Autodesk Inventor part; units mm, degrees
ref_plane "Work Plane1" through (0, 0, 22) normal (0, 0, 1) x (1, 0, 0)
ref_plane "Plano de trabajo2" through (0, 0, 54) normal (0, 0, 1) x (1, 0, 0)
ref_plane "YZ Plane" through (0, 0, 0) normal (1, 0, 0) x (0, 1, 0)
sketch "Sketch1" plane through (0, 0, 0) normal (0, 0, 1) x (1, 0, 0)
  circle A0 centre (0, 0) radius 50
  circle A1 centre (0, 0) radius 12.5
  circle A2 centre (0, 0) radius 14.5
  line L0 (-15.5, -15.5) -> (15.5, -15.5) construction
  line L1 (15.5, -15.5) -> (15.5, 15.5) construction
  line L2 (15.5, 15.5) -> (-15.5, 15.5) construction
  line L3 (-15.5, 15.5) -> (-15.5, -15.5) construction
  line L4 (-15.5, -15.5) -> (15.5, 15.5) construction
  line L5 (15.5, -15.5) -> (-15.5, 15.5) construction
  dimension "Diametro" = 100
  dimension "d1" = 25
  dimension "d2" = 2
  dimension "d8" = 31
extrude "Extrusion1" add sketch "Sketch1" along normal blind 7 contours A0 | A2
extrude "Extrusion2" add sketch "Sketch1" along normal blind 100 contours A2
ref_plane "Work Plane1" through (0, 0, 22) normal (0, 0, 1) x (1, 0, 0)
sketch "Sketch2" plane through (0, 0, 22) normal (0, 0, 1) x (1, 0, 0)
  arc A0 (2.5, 24.8747) -> (-2.5, 24.8747) centre (0, 0) ccw
  line L0 (2.5, 24.8747) -> (2.5, 14.2829)
  line L1 (-2.5, 24.8747) -> (-2.5, 14.2829)
  line L2 (0, -70) -> (0, 70)
  circle A1 centre (0, 0) radius 14.5
  point P0 (0, 25)
  dimension "d24" = 5
  dimension "d25" = 25
  dimension "Dedos" = 5
extrude "Extrusion3" add sketch "Sketch2" along normal blind 15 contours L0 A1 L2 A0 | L2 A1 L1 A0
sketch "Sketch3" plane through (0, 0, 0) normal (1, 0, 0) x (0, 1, 0)
  line L0 (25, 37) -> (24.8747, 37)
  line L1 (14.2829, 22) -> (14.5, 22)
  line L2 (25, 22) -> (25, 37)
  line L3 (14.2829, 22) -> (14.2829, 37)
  circle A0 centre (25.74, 29.5) radius 1.5
  line L4 (0, -7.4) -> (0, 44.4)
  point P0 (0, 0)
  point P1 (25, 29.5)
  dimension "d31" = 3
  dimension "d92" = 25.74
fillet "Fillet2" radius 8 1 edges at (0, 25, 22)
pattern_circular "Circular Pattern1" count 4 over 360 about axis through (0, 0, 0) along (0, 0, 1) of "Fillet2", "Extrusion3"
ref_plane "Plano de trabajo2" through (0, 0, 54) normal (0, 0, 1) x (1, 0, 0)
sketch "Boceto4" plane through (0, 0, 54) normal (0, 0, 1) x (1, 0, 0)
  circle A0 centre (0, 0) radius 17.5
  circle A1 centre (0, 0) radius 14.5
  line L0 (4, -23.75) -> (4, -26.75)
  dimension "d54" = 35
extrude "Extrusión5" add sketch "Boceto4" against normal up to surface (47 mm away)
sketch "Boceto5" plane through (0, 0, 37) normal (0, 0, 1) x (0, 1, 0)
  arc A0 (-2.5, -17.3205) -> (2.5, -17.3205) centre (0, 0) ccw
  line L0 (-2.5, -17.3205) -> (-2.5, -24.8747)
  arc A1 (-2.5, -24.8747) -> (2.5, -24.8747) centre (0, 0) ccw
  line L1 (2.5, -24.8747) -> (2.5, -17.3205)
  circle A2 centre (0, 0) radius 14.5
  line L2 (2.5, -17.3205) -> (2.5, -14.2829)
  line L3 (-2.5, -17.3205) -> (-2.5, -14.2829)
extrude "Extrusión6" add sketch "Boceto5" along normal blind 20 contours L3 A2 L2 A0 | A0 L1 A1 L0
fillet "Empalme4" radius 8 1 edges at (25, 0, 57)
pattern_circular "Patrón circular2" count 4 over 360 about axis through (0, 0, 54) along (0, 0, -1) of "Extrusión6", "Empalme4"
chamfer "Chaflán1" distance 2 angle 45 1 edges at (-14.5, 0, 100)
sketch "Boceto6" plane through (0, 0, 7) normal (0, 0, 1) x (1, 0, 0)
  circle A0 centre (0, 0) radius 50
  arc A1 (17.3205, 2.5) -> (2.5, 17.3205) centre (0, 0) ccw construction
  line L0 (0, 0) -> (32.476, 18.75) construction
  arc A2 (17.3205, 2.5) -> (2.5, 17.3205) centre (0, 0) ccw construction
  point P0 (16.25, -6.4952)
  point P1 (16.25, 6.4952)
  point P2 (0, 37.5)
  point P3 (-32.476, 18.75)
  point P4 (-32.476, -18.75)
  point P5 (0, -37.5)
  point P6 (32.476, -18.75)
  point P7 (10.8253, 13.75)
  point P8 (15.1554, 8.75)
  dimension "d73" = 360
  dimension "d91" = 37.5
sketch "Boceto8" plane through (0, 0, 7) normal (0, 0, 1) x (1, 0, 0)
  circle A0 centre (0, 0) radius 17.5
  circle A1 centre (0, 0) radius 50
  circle A2 centre (0, 0) radius 46
  dimension "Espesor" = 4
extrude "Extrusión8" add sketch "Boceto8" along normal blind 6 contours A2
sketch "Boceto9" plane through (2.5, 14.0104, 54) normal (1, 0, 0) x (0, -1, 0)
  line L0 (16.5104, 0) -> (28.2932, 0)
  line L1 (-35.9896, 54) -> (64.0104, 54)
  point P0 (1.4018, 24.5)
  point P1 (22.4018, 0)
  dimension "d124" = 21
  dimension "d125" = 29.5
hole "Agujero4" at (2.5, 12.6086, 29.5) direction (-1, 0, 0) diameter 3.4 depth 5
pattern_circular "Patrón circular3" count 4 over 360 about axis through (0, 0, 54) along (0, 0, -1) of "Agujero4"
sketch "Boceto13" plane through (0, 0, 13) normal (0, 0, 1) x (1, 0, 0)
  point P0 (0, 0)
sketch "Boceto15" plane through (0, 0, 0) normal (0, 0, -1) x (-1, 0, 0)
  circle A0 centre (0, 0) radius 27.5 construction
  point P0 (27.5, 0)
  point P1 (13.75, 23.8157)
  point P2 (-13.75, 23.8157)
  point P3 (-27.5, 0)
  point P4 (-13.75, -23.8157)
  point P5 (13.75, -23.8157)
  dimension "d134" = 55
  dimension "d137" = 360
hole "Agujero8" at (-13.75, -23.8157, 0) at (13.75, -23.8157, 0) at (27.5, 0, 0) at (13.75, 23.8157, 0) at (-13.75, 23.8157, 0) at (-27.5, 0, 0) direction (0, 0, 1) diameter 3.4 end through all
sketch "Boceto16" plane through (0, 0, 0) normal (0, 0, -1) x (-1, 0, 0)
  circle A0 centre (0, 0) radius 32.465
  dimension "d146" = 64.93
extrude "Extrusión10" cut sketch "Boceto16" against normal blind 8
sketch "Boceto18" plane through (0, 0, 0) normal (0, 0, -1) x (-1, 0, 0)
  point P0 (0, 0)
  point P1 (-41.233, 0)
  point P2 (-29.1561, -29.1561)
  point P3 (0, -41.233)
  point P4 (29.1561, -29.1561)
  point P5 (41.233, 0)
  point P6 (29.1561, 29.1561)
  point P7 (0, 41.233)
  point P8 (-29.1561, 29.1561)
  dimension "d162" = 41.233
  dimension "d165" = 360
hole "Agujero10" at (41.233, 0, 0) at (29.1561, -29.1561, 0) at (0, -41.233, 0) at (-29.1561, -29.1561, 0) at (-41.233, 0, 0) at (-29.1561, 29.1561, 0) at (0, 41.233, 0) at (29.1561, 29.1561, 0) direction (0, 0, 1) diameter 2.459 depth 10
sketch "Sketch19" plane through (14.2829, -2.5, 54) normal (0, -1, 0) x (1, 0, 0)
  circle A0 centre (6.7167, -24.5) radius 1.7
  line L0 (3.0377, 0) -> (3.0377, -31.9844)
  line L1 (3.0377, 0) -> (-11.7829, 0)
  point P0 (-14.2829, -54)
  dimension "d174" = 3.4
  dimension "d175" = 3.679
  dimension "d176" = 24.5
hole "Hole11" at (20.9995, -2.5, 29.5) direction (0, 1, 0) diameter 4 depth 5
pattern_circular "Circular Pattern4" count 4 over 360 about axis through (0, 0, 0) along (0, 0, 1) of "Hole11"
sketch "Sketch20" plane through (0, 0, 13) normal (0, 0, 1) x (1, 0, 0)
  circle A0 centre (-27.5, 0) radius 1.7
  circle A1 centre (-13.75, 23.8157) radius 1.7
  circle A2 centre (13.75, 23.8157) radius 1.7
  circle A3 centre (27.5, 0) radius 1.7
  circle A4 centre (13.75, -23.8157) radius 1.7
  circle A5 centre (-13.75, -23.8157) radius 1.7
  circle A6 centre (0, 0) radius 46
  circle A7 centre (0, 0) radius 17.5
  circle A8 centre (0, 0) radius 46
extrude "Extrusion12" cut sketch "Sketch20" along normal up to surface contours A6 | A7
sketch "Sketch21" plane through (0, 0, 13) normal (0, 0, 1) x (1, 0, 0)
  circle A0 centre (0, 0) radius 12.5
  circle A1 centre (-27.5, 0) radius 1.7
  circle A2 centre (-13.75, 23.8157) radius 1.7
  circle A3 centre (13.75, 23.8157) radius 1.7
  circle A4 centre (27.5, 0) radius 1.7
  circle A5 centre (13.75, -23.8157) radius 1.7
  circle A6 centre (-13.75, -23.8157) radius 1.7
  circle A7 centre (0, 0) radius 46
  circle A8 centre (-13.75, 23.8157) radius 1.7
  circle A9 centre (13.75, -23.8157) radius 1.7
extrude "Extrusion13" add sketch "Sketch21" against normal up to surface (5 mm away) contours A2 | A5
equation "\"d24\" = Dedos"
equation "\"d91\" = 0.375 * Diametro"
properties part number "Soporte2" material "Aluminum 7075"
Build history of the part. All positions in model axes, mm. A direction names the side the tool comes from. Round coordinates to 2 decimals unless told otherwise and drop trailing zeros. Write each loop counter-clockwise with the first axis right and the second up, starting at its lowest first coordinate (ties: lowest second). Pieces come first, ordered by that corner, then holes. Notation, with made-up numbers: (-31, -7.75) - (1, -7.75) arc R29 cw to (1, 14.25) - close; hole circle Ø5 at (43.5, -16.5). An arc over 180 degrees is marked (long way). One line per question, with ' | ' between items.
1. Band-saw the part on D-D, the plane y = 14.5. Write the cut outline in (x, z).
Results are:
outline: (-47.85, 0) - (-29.05, 0) - (-29.05, 8) - (29.05, 8) - (29.05, 0) - (47.85, 0) - (47.85, 7) - (43.65, 7) - (43.65, 13) - (-43.65, 13) - (-43.65, 7) - (-47.85, 7) - close
2. Band-saw the part on B-B, the plane x = 0. Write the cut outline in (y, z) (1 decimal).
Results are:
outline: (-50, 0) - (-42.5, 0) - (-42.5, 10) - (-40, 10) - (-40, 0) - (-32.5, 0) - (-32.5, 8) - (-12.5, 8) - (-12.5, 13) - (-46, 13) - (-46, 7) - (-50, 7) - close; (12.5, 8) - (32.5, 8) - (32.5, 0) - (40, 0) - (40, 10) - (42.5, 10) - (42.5, 0) - (50, 0) - (50, 7) - (46, 7) - (46, 13) - (12.5, 13) - close
3. Tool access for faces 4 (the face through (29.63, 30.29, 5.07)), 5 (the face through (13.675, 22.117, 10.535)): list every direction of +Z, -Z, +X, -X, +Y, -Y with a clear straight run to the whole face (end or side of a thin tool).
Results are:
face 4: -Z | face 5: +Z, -Z
4. Drill centre lines: line 1 along X through (y, z) = (1, 3); line 2 along X through (y, z) = (-0.5, 11.5); line 3 along Z through (x, y) = (-28, 11.5). Where is each one in solid material? Low to high. Write a range as from..to.
Results are:
line 1: -49.99..-41.95, -40.52..-32.45, 32.45..40.52, 41.95..49.99 | line 2: -46..-29.12, -25.88..-12.49, 12.49..25.88, 29.12..46 | line 3: 8..13
5. Band-saw the part on C-C, the plane z = 1.5. Give the number of separate pieces and of enclosed holes in the cut face, and give its area (3 significant figures).
Results are:
separate pieces: 1 | enclosed holes: 9 | area: 4,500 mm^2
6. Drop flat-ended pins along their axis: pin 1 Ø1 at (x, z) = (19.5, 2.5) entering from +Y; pin 2 Ø6 at (x, z) = (11, 6.5) entering from -Y; pin 3 Ø1.2 at (x, y) = (41, 0.5) entering from -Z. Give the stop position or say it passes through.
Results are:
pin 1: y = 46.25 | pin 2: y = -49.36 | pin 3: z = 10
7. Band-saw the part on A-A, the plane z = 11.25. Write the cut outline in (x, y).
Results are:
outline: circle Ø92 at (0, 0); hole circle Ø3.4 at (-27.5, 0); hole circle Ø3.4 at (-13.75, -23.82); hole circle Ø25 at (0, 0); hole circle Ø3.4 at (13.75, 23.82); hole circle Ø3.4 at (27.5, 0)
8. Mould opens along X. For faces 1 (the face through (47.69, -15.02, 3.45)), 2 (the face through (-28.7, 30.3, 5.1)), 3 (the face through (10, -10, 13)) say: released by +X, released by -X, zero draft, split by the parting line, or undercut.
Results are:
face 1: split by the parting line | face 2: undercut | face 3: zero draft
